Verification items for the finished model (mm, model axes). A direction names the side the tool comes from. Give positions to 0.01 mm unless a question says otherwise; leave off trailing zeros. Loops run counter-clockwise (first coordinate to the right, second up) from the corner with the lowest first, then second, coordinate; pieces in that order, holes last. Notation, with made-up numbers: (86.25, 21) -> (121.25, 21) arc R25 cw to (121.25, 52) -> close; hole circle Ø5 at (75, 73.5). An arc over 180 degrees is marked (long way). Answer in a Markdown table with one row per item. Add a question column.
Q1. Section check D-D on z = 6.5. Enter the section's corners in (x, y).
Q2. Section check C-C on y = 3.5. Enter the section's corners in (x, z), and give its area (4 significant figures).
Q3. Release check for a two-part mould opening along Y. For faces 1 (the face through (11, 0, 8)), 2 (the face through (12, 7, 11)), 3 (the face through (12.029, 2.906, 19.432)), 4 (the face through (1.95, 3.57, 1.52)) record: pulls with the +Y half, pulls with the -Y half, needs draft (parallel to the pull), parting line crosses it, or undercut.
Q4. Material ranges on probe 1 along Y at (x, z) = (12.1, 18); probe 2 along Y at (x, z) = (3.5, 2.2); probe 3 along Z at (x, y) = (3, 9), recorded low to high.
Q5. Section check A-A on z = 18. Enter the section's corners in (x, y).
Q6. Set-up check for faces 5 (the face through (4, 8, 3)), 6 (the face through (3, 15.6, 13)), 7 (the face through (10.55, 3, 13)), 8 (the face through (3, 17, 23)), 9 (the face through (7, 16, 9)): record each of +Z, -Z, +X, -X, +Y, -Y from which the full face is reachable in a straight line by a thin tool's end or side.
Q7. Gauge pin test, flat ends, axial feed: P1, Ø6, axis at y = 10.5, z = 13.5, coming from the +X side; P2, Ø6, axis at x = 11.5, z = 6.5, coming from the +Y side; P3, Ø8, axis at x = 1.5, y = 8.5, coming from the +Z side; P4, Ø7.5, axis at y = 3.5, z = 17, coming from the -X side. Record the tip position at first contact, or that the pin passes through.
Q8. Section check B-B on x = 3.5. Enter the section's corners in (y, z), and give its area (3 significant figures).
```python
from build123d import *

# Parameters (mm, degrees)
ESQUISSE1_W             = 7
ESQUISSE1_H             = 11.6
ESQUISSE1_H_2           = 7
ESQUISSE1_W_2           = 6.55
BOSS_EXTRU_1_DEPTH      = 3
ESQUISSE2_W             = 7
ESQUISSE2_H             = 3
BOSS_EXTRU_2_DEPTH      = 20
ESQUISSE3_W             = 3
ESQUISSE3_H             = 7
BOSS_EXTRU_3_DEPTH      = 20
ESQUISSE4_R             = 1.55
ENL_V_MAT_EXTRU_1_DEPTH = 20
ESQUISSE5_R             = 1.55
ENL_V_MAT_EXTRU_2_DEPTH = 20
ESQUISSE6_R             = 1.55
ENL_V_MAT_EXTRU_3_DEPTH = 20


with BuildPart() as part:
    # Esquisse1 → Boss.-Extru.1 (new body)
    with BuildSketch(Plane.XY):
        with Locations((3.5, 12.8)):
            Rectangle(ESQUISSE1_W, ESQUISSE1_H)
        with Locations((3.5, 3.5)):
            Rectangle(ESQUISSE1_W, ESQUISSE1_H_2)
        with Locations((10.275, 3.5)):
            Rectangle(ESQUISSE1_W_2, ESQUISSE1_H_2)
    extrude(amount=BOSS_EXTRU_1_DEPTH)

    # Esquisse2 → Boss.-Extru.2 (add)
    with BuildSketch(Plane.XY.offset(3)):
        with Locations((3.5, 17.1)):
            Rectangle(ESQUISSE2_W, ESQUISSE2_H)
    extrude(amount=BOSS_EXTRU_2_DEPTH)

    # Esquisse3 → Boss.-Extru.3 (add)
    with BuildSketch(Plane.XY.offset(3)):
        with Locations((12.05, 3.5)):
            Rectangle(ESQUISSE3_W, ESQUISSE3_H)
    extrude(amount=BOSS_EXTRU_3_DEPTH)

    # Esquisse4 → Enlèv. mat.-Extru.1 (cut)
    with BuildSketch(Plane.XZ.offset(-15.6)):
        with Locations(Location((3.5, 10.35, 0), (0, 0, 270))):
            Circle(ESQUISSE4_R)
    extrude(amount=-ENL_V_MAT_EXTRU_1_DEPTH, mode=Mode.SUBTRACT)

    # Esquisse5 → Enlèv. mat.-Extru.2 (cut)
    with BuildSketch(Plane.ZY.offset(-10.55)):
        with Locations((18, 3.5)):
            Circle(ESQUISSE5_R)
    extrude(amount=-ENL_V_MAT_EXTRU_2_DEPTH, mode=Mode.SUBTRACT)

    # Esquisse6 → Enlèv. mat.-Extru.3 (cut)
    with BuildSketch(Plane.XY.offset(3)):
        with Locations((3.5, 3.5)):
            Circle(ESQUISSE6_R)
    extrude(amount=-ENL_V_MAT_EXTRU_3_DEPTH, mode=Mode.SUBTRACT)


solid = part.part
```
Taken from the geometry:
| question | item | result |
|---|---|---|
| 1 | outline | (0, 15.6) -> (7, 15.6) -> (7, 18.6) -> (0, 18.6) -> close; (10.55, 0) -> (13.55, 0) -> (13.55, 7) -> (10.55, 7) -> close |
| 2 | outline | (0, 0) -> (1.95, 0) -> (1.95, 3) -> (0, 3) -> close; (5.05, 0) -> (13.55, 0) -> (13.55, 16.45) -> (10.55, 16.45) -> (10.55, 3) -> (5.05, 3) -> close; (10.55, 19.55) -> (13.55, 19.55) -> (13.55, 23) -> (10.55, 23) -> close |
| 2 | area | 82.05 mm² |
| 3 | face 1 | pulls with the -Y half |
| 3 | face 2 | pulls with the +Y half |
| 3 | face 3 | undercut |
| 3 | face 4 | undercut |
| 4 | probe 1 | y = 0 to 1.95, 5.05 to 7 |
| 4 | probe 2 | y = 0 to 1.95, 5.05 to 18.6 |
| 4 | probe 3 | z = 0 to 3 |
| 5 | outline | (0, 15.6) -> (7, 15.6) -> (7, 18.6) -> (0, 18.6) -> close; (10.55, 0) -> (13.55, 0) -> (13.55, 1.95) -> (10.55, 1.95) -> close; (10.55, 5.05) -> (13.55, 5.05) -> (13.55, 7) -> (10.55, 7) -> close |
| 6 | face 5 | +Z, -X, -Y |
| 6 | face 6 | +Z, +X, -X, -Y |
| 6 | face 7 | +Z, -X, +Y, -Y |
| 6 | face 8 | +Z, +X, -X, +Y, -Y |
| 6 | face 9 | +Z, -Z, +X, +Y |
| 7 | P1 | passes through |
| 7 | P2 | stops at y = 7 |
| 7 | P3 | stops at z = 3 |
| 7 | P4 | stops at x = 10.55 |
| 8 | outline | (0, 0) -> (1.95, 0) -> (1.95, 3) -> (0, 3) -> close; (5.05, 0) -> (18.6, 0) -> (18.6, 8.8) -> (15.6, 8.8) -> (15.6, 3) -> (5.05, 3) -> close; (15.6, 11.9) -> (18.6, 11.9) -> (18.6, 23) -> (15.6, 23) -> close |
| 8 | area | 97.2 mm² |
